For this review, use the dimensioned drawing (mm, ordinates from the lowest corner) and the shaded views. A direction names the side the tool comes from. Give positions to 0.01 mm unless a question says otherwise; leave off trailing zeros. Order: outer loops, then holes, each group sorted by start corner. A loop starts at its lowest first (then second) coordinate and runs counter-clockwise, first axis right, second up. Notation, with made-up numbers: M 39.25,69 L 73.25,69 A21 cw 73.25,77 Z; hole C 66.5,75.25 d6. An arc over 180 degrees is marked long. Use CSV: the item, a comma, the result in double quotes. Start each with the question number.
(1) Consider section C-C (x = 31). Write out the cut boundary in (y, z).
(2) Consider section D-D (y = 18.5). Write out the cut boundary in (x, z).
(3) Consider section B-B (z = 10). Write out the cut boundary in (x, y) (1 decimal), and give its area (3 significant figures).
(4) Wall thickness on L1, parallel to Y at x = 6.5, z = 16; L2, parallel to Z at x = 50.5, y = 22; L3, parallel to X at y = 20, z = 42.5: over which ranges is each line inside the solid? List them lowest first. Write a range as from..to.
(5) Tool access review of the marked faces 4, 5, 6 and 7: name each direction out of +Z, -Z, +X, -X, +Y, -Y from which nothing blocks a thin tool from reaching the whole face with its end or side.
(6) Consider section A-A (y = 37). Write out the cut boundary in (x, z) (1 decimal).
(7) Draft analysis for pull direction Y (two halves, no side actions). For the marked faces 1, 2 and 3, state which applies: pulls with the +Y half, pulls with the -Y half, needs draft (parallel to the pull), parting line crosses it, or undercut.
(8) Clearance check with flat-ended pins moving along their axes: P1, Ø16.5, axis at x = 53, y = 36, coming from the -Z side; P2, Ø2, axis at x = 30, y = 38.5, coming from the -Z side; P3, Ø6, axis at y = 30.5, z = 20.5, coming from the -X side; P4, Ø5, axis at y = 15.5, z = 29.5, coming from the -X side. State where each tip first meets the part, or that it passes through.
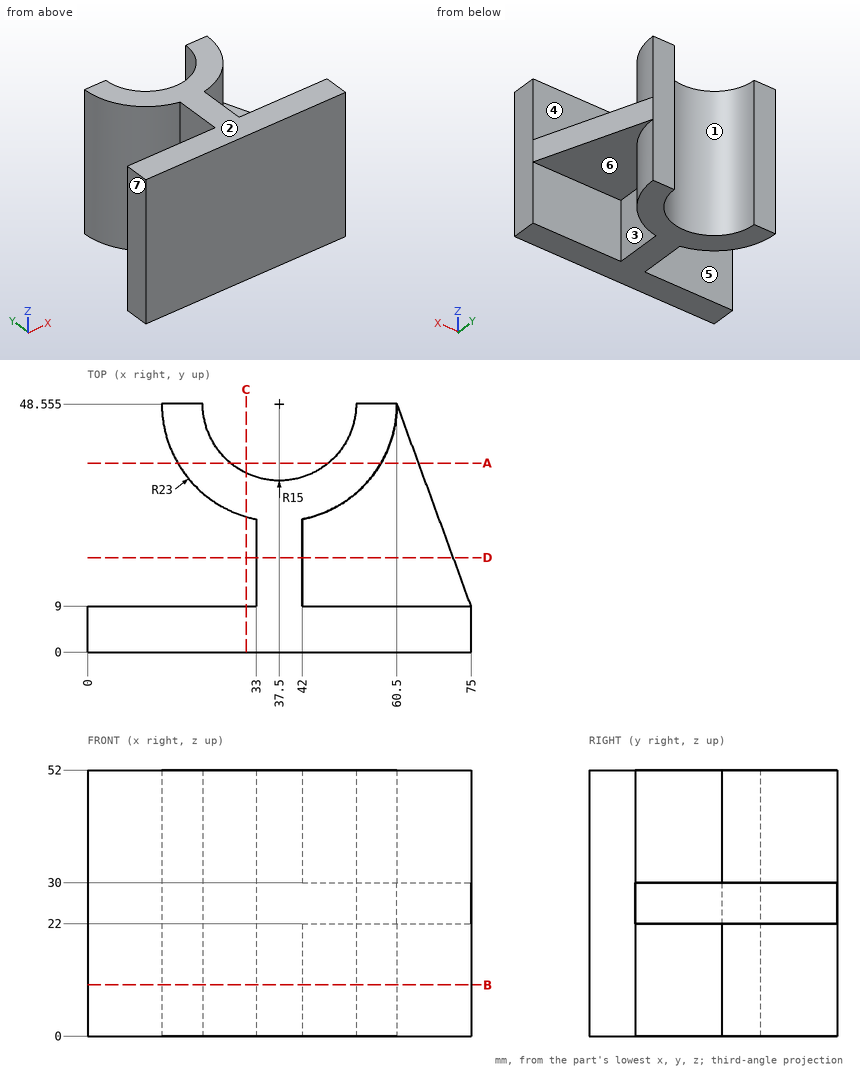
Check result:
1,outline,"M 0,0 L 9,0 L 9,52 L 0,52 Z; M 26.49,0 L 35.04,0 L 35.04,52 L 26.49,52 Z"
2,outline,"M 33,0 L 42,0 L 42,22 L 71.52,22 L 71.52,30 L 42,30 L 42,52 L 33,52 Z"
3,outline,"M 0,0 L 75,0 L 75,9 L 42,9 L 42,26 A23 ccw 60.5,48.6 L 52.5,48.6 A15 cw 22.5,48.6 L 14.5,48.6 A23 ccw 33,26 L 33,9 L 0,9 Z"
3,area,"1,300 mm^2"
4,L1,"y = 0..9"
4,L2,"z = 22..30"
4,L3,"x = 33..42"
5,face 4,"+Z, +X"
5,face 5,"+Z, -Z, -X"
5,face 6,"-Z, +X"
5,face 7,"+Z, -Z, -X, +Y, -Y"
6,outline,"M 17.6,0 L 27.9,0 L 27.9,52 L 17.6,52 Z; M 47.1,0 L 57.4,0 L 57.4,22 L 64.7,22 L 64.7,30 L 57.4,30 L 57.4,52 L 47.1,52 Z"
7,face 1,"pulls with the +Y half"
7,face 2,"needs draft"
7,face 3,"undercut"
8,P1,"stops at z = 0"
8,P2,"passes through"
8,P3,"stops at x = 20.11"
8,P4,"stops at x = 33"
